Could you check a few things on this model? Use its own coordinates, in mm. Face numbers are marked on the shaded views. A direction names the side the tool comes from. Give positions to 0.01 mm unless a question says otherwise; leave off trailing zeros. Order: outer loops, then holes, each group sorted by start corner. A loop starts at its lowest first (then second) coordinate and runs counter-clockwise, first axis right, second up.
(1) Imagine slicing it at D-D, the plane z = 1. Write out the boundary of the cut face in (x, y).
(2) Will these pins go through, and if not, where does the flat tip stop? pin 1 (4 mm diameter, centred on x = 11.5, z = 3, fed in from -Y); pin 2 (7.5 mm diameter, centred on x = 12, y = 12.5, fed in from +Z); pin 3 (1 mm diameter, centred on x = 28, z = 5.5, fed in from +Y).
(3) Imagine slicing it at A-A, the plane z = 8.5. Write out the boundary of the cut face in (x, y), then the cut area to 3 significant figures.
(4) If I drill on probe 1 along Z at (x, y) = (10.5, 4.5); probe 2 along X at (y, z) = (4, 4); probe 3 along Y at (x, z) = (23, 3.5), over which ranges is the centre line in solid material (lowest first)?
(5) Imagine slicing it at C-C, the plane x = 44. Write out the boundary of the cut face in (y, z).
(6) Imagine slicing it at B-B, the plane y = 5.5. Write out the boundary of the cut face in (x, z) (3 decimals).
(7) On a 3-axis mill with a long thin cutter (end or side, diameter ignored), from which of +Z, -Z, +X, -X, +Y, -Y can I reach the whole of each face in a straight line? I mean the marked faces 1, 2 and 3. Say none if no direction works.
(8) If we mould it in two halves opening along X, with no side actions, what happens to the marked faces 4, 5 and 6? For each: released by +X, released by -X, zero draft, split by the parting line, or undercut.
Autodesk Inventor part; units mm, degrees
ref_plane "YZ Plane" through (0, 0, 0) normal (1, 0, 0) x (0, 1, 0)
ref_plane "XZ Plane" through (0, 0, 0) normal (0, 1, 0) x (-1, 0, 0)
ref_plane "XY Plane" through (0, 0, 0) normal (0, 0, 1) x (1, 0, 0)
sketch "Base Sketch" plane through (0, 0, 0) normal (0, 0, 1) x (1, 0, 0)
  line L0 (22, 0) -> (0, 0)
  line L1 (3.4939, 2.3817) -> (36.1282, 24.6282)
  line L2 (41, 20) -> (22, 0)
  line L3 (41, 20) -> (85.6646, 14.5159)
  line L4 (90.1222, 17.9986) -> (36.1282, 24.6282)
  line L5 (36.1282, 24.6282) -> (41, 20) construction
  line L6 (41, 20) -> (41.4875, 23.9702)
  line L7 (3.4939, 2.3817) -> (0, 0) construction
  line L8 (0, 0) -> (0, -2.6652) construction
  arc A0 (3.4939, 2.3817) -> (0, -4.2285) centre (8, -4.2285) ccw
  line L9 (85.6646, 14.5159) -> (79.693, -34.1189)
  line L10 (79.693, -34.1189) -> (83.6632, -34.6064)
  line L11 (83.6632, -34.6064) -> (90.1222, 17.9986)
  point P0 (1.2088, 0)
  dimension "d2" = 22
  dimension "d3" = 20
  dimension "d4" = 19
  dimension "d5" = 4
  dimension "d24" = 8
  dimension "d25" = 4
  dimension "d27" = 7
  dimension "d28" = 45
  dimension "d29" = 49
extrude "Lower Arm" add sketch "Base Sketch" along normal blind 5.25 contours L0 A0 L1 L4 L6 L2
extrude "Upper Arm" add sketch "Base Sketch" along normal blind 10.5 contours L6 L4 L11 L10 L9 L3
fillet "Fillet1" radius 8 2 edges at (36.1282, 24.6282, 2.625) (90.1222, 17.9986, 5.25)
fillet "Fillet1" radius 4 1 edges at (85.6646, 14.5159, 5.25)
fillet "Fillet3" radius 6 1 edges at (83.6632, -34.6064, 5.25)
fillet "Fillet4" radius 0.4 1 edges at (79.693, -34.1189, 5.25)
equation "\"d2\" = ConnectionWidth"
equation "\"d3\" = ArmDistance"
equation "\"d4\" = ArmTravelToDistance"
equation "\"d5\" = ArmThickness"
equation "\"d25\" = ArmThickness"
equation "\"d18\" = 0.5 * KeySpacing + 0.5 * KeyWidth"
equation "\"d20\" = KeyWidth + KeySpacing"
properties part number "HousingArm0" material "PLA Plastic (Glacial Blue)"
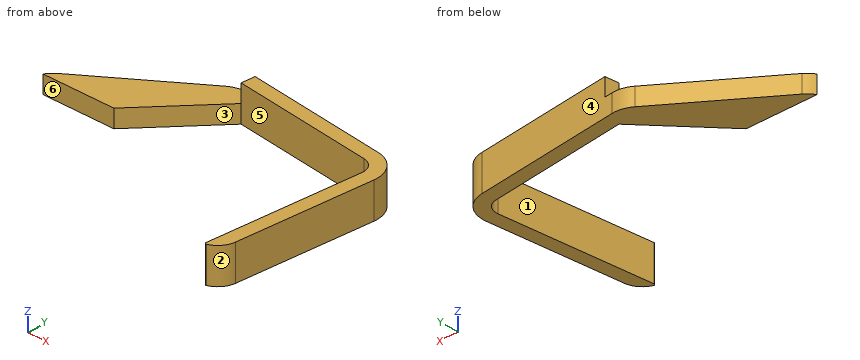
Answer block:
1. outline: (1.21, 0) - (22, 0) - (41, 20) - (81.69, 15) arc R4 cw to (85.18, 10.55) - (79.77, -33.53) arc R0.4 ccw to (80.29, -33.95) arc R6 ccw to (84.35, -28.99) - (89.15, 10.06) arc R8 ccw to (82.18, 18.97) - (39.12, 24.26) arc R8 ccw to (33.64, 22.93) - (3.49, 2.38) arc R8 ccw to start
2. pin 1: stops at y = 0
2. pin 2: stops at z = 5.25
2. pin 3: stops at y = 19.38
3. outline: (41, 20) - (81.69, 15) arc R4 cw to (85.18, 10.55) - (79.77, -33.53) arc R0.4 ccw to (80.29, -33.95) arc R6 ccw to (84.35, -28.99) - (89.15, 10.06) arc R8 ccw to (82.18, 18.97) - (41.49, 23.97) - close
3. area: 375 mm2
4. probe 1: z = 0 to 5.25
4. probe 2: x = 5.87 to 25.8, 84.37 to 88.4
4. probe 3: y = 1.05 to 15.68
5. outline: (19.63, 0) - (23.66, 0) - (23.66, 10.5) - (19.63, 10.5) - close
6. outline: (8.068, 0) - (27.225, 0) - (27.225, 5.25) - (8.068, 5.25) - close; (84.558, 0) - (88.588, 0) - (88.588, 10.5) - (84.558, 10.5) - close
7. face 1: +Z, -Z
7. face 2: +Z, -Z, +X, -Y
7. face 3: +Z, -Z, -Y
8. face 4: released by +X
8. face 5: undercut
8. face 6: zero draft
